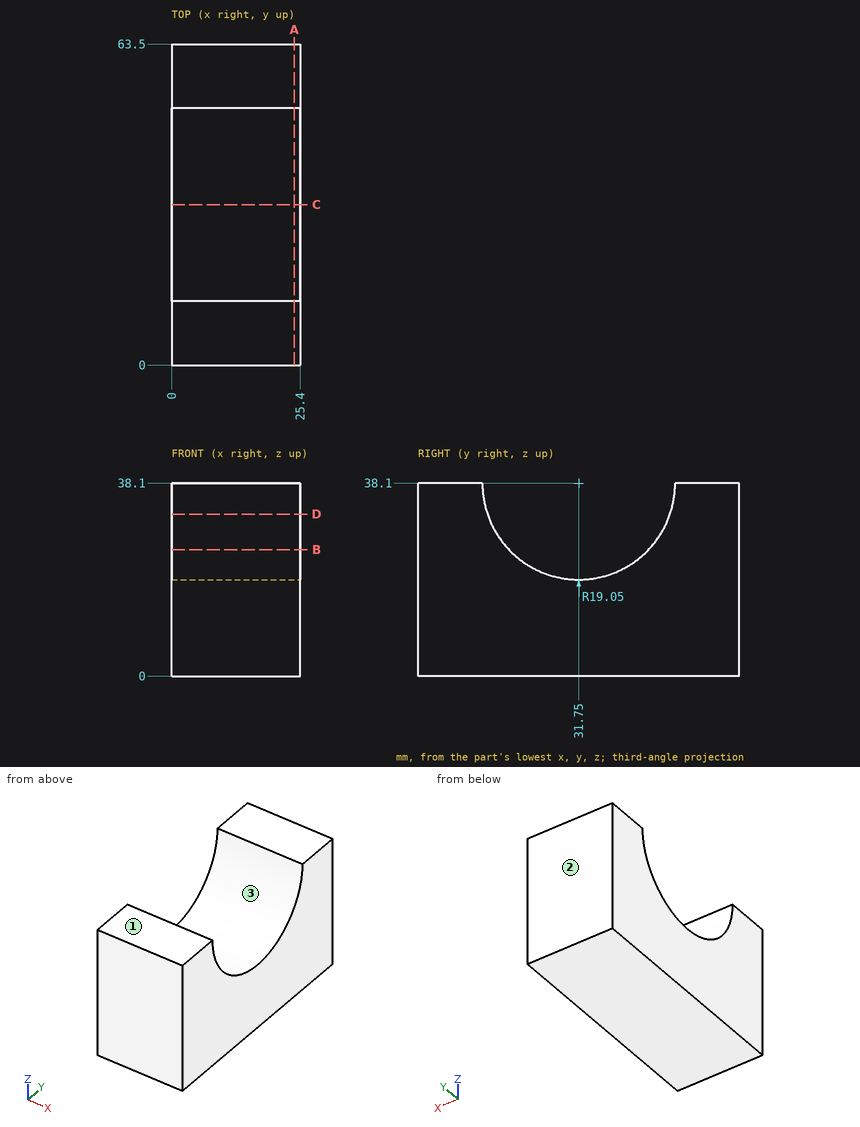
Source: three-view drawing plus pictorial views. Frame: mm from the lowest corner of the part. Round coordinates to 2 decimals unless told otherwise and drop trailing zeros. Order: outer loops, then holes, each group sorted by start corner. A loop starts at its lowest first (then second) coordinate and runs counter-clockwise, first axis right, second up. Notation, with made-up numbers: (60, 74) - (81, 74) arc R23 cw to (81, 86) - close; hole circle Ø6 at (43.25, 55.25). An arc over 180 degrees is marked (long way). Answer in a Markdown table with one row per item.
Item 1: Section query C-C (y = 31.75). Return the cut outline in (x, z), then the cut area to 3 significant figures.
Model answer:
| item | result |
|---|---|
| outline | (0, 0) - (25.4, 0) - (25.4, 19.05) - (0, 19.05) - close |
| area | 484 mm² |
Item 2: Mould query, pull axis Y, two halves, no side actions, for the marked faces 1, 2 and 3. Classes: released by +Y, released by -Y, zero draft, split by the parting line, or undercut.
Model answer:
| item | result |
|---|---|
| face 1 | zero draft |
| face 2 | released by +Y |
| face 3 | undercut |
Item 3: Pin query (flat end, axial travel): pin 1 (2 mm diameter, centred on x = 22, y = 25, fed in from +Z). Return the tip coordinate at first contact, or that it passes through.
Model answer:
| item | result |
|---|---|
| pin 1 | stops at z = 20.7 |
Item 4: Section query B-B (z = 25). Return the cut outline in (x, y).
Model answer:
| item | result |
|---|---|
| outline | (0, 0) - (25.4, 0) - (25.4, 17.92) - (0, 17.92) - close; (0, 45.58) - (25.4, 45.58) - (25.4, 63.5) - (0, 63.5) - close |
Item 5: Section query D-D (z = 32). Return the cut outline in (x, y).
Model answer:
| item | result |
|---|---|
| outline | (0, 0) - (25.4, 0) - (25.4, 13.7) - (0, 13.7) - close; (0, 49.8) - (25.4, 49.8) - (25.4, 63.5) - (0, 63.5) - close |
Item 6: Section query A-A (x = 24.25). Return the cut outline in (y, z), then the cut area to 3 significant figures.
Model answer:
| item | result |
|---|---|
| outline | (0, 0) - (63.5, 0) - (63.5, 38.1) - (50.8, 38.1) arc R19.05 cw to (12.7, 38.1) - (0, 38.1) - close |
| area | 1,850 mm² |
Item 7: Line query: line 1 (Y direction, x = 23, z = 28.5); line 2 (Y direction, x = 11.5, z = 22); line 3 (Z direction, x = 18, y = 38). Output: solid intervals per line, ascending.
Model answer:
| item | result |
|---|---|
| line 1 | y = 0 to 15.3, 48.2 to 63.5 |
| line 2 | y = 0 to 21.57, 41.93 to 63.5 |
| line 3 | z = 0 to 20.1 |
